from build123d import *

# Parameters (mm, degrees)
EXTRUDE023_DEPTH                          = 4
EXTRUDE022_DEPTH                          = 4
EXTRUDE022_ONTO_SKETCH021_PLACEMENT_ANGLE = 120


with BuildPart() as extrude023:
    # Sketch022 (on Face6 of Extrude022) → Extrude023 (new body)
    with BuildSketch(Plane(origin=(26.5, 0, 0), x_dir=(0, -1, 0), z_dir=(-1, 0, 0))):
        Polygon((-15.99404, 23.43698), (-11, 10), (-19, 10), (-22.458142, 20.240827), align=None)
    extrude(amount=-EXTRUDE023_DEPTH)


with BuildPart() as pin_boot:
    # Sketch021 as drawn → Extrude022 (new)
    with BuildSketch(Plane.XY):
        Polygon((29, 44.3), (33, 44.3), (33, 18.3), (30.5, 12.3), (30.5, 6.3), (26.5, 6.3), (26.5, 12.3), (29, 18.3), align=None)
    extrude(amount=EXTRUDE022_DEPTH)


with BuildPart() as pin_boot_1:
    # Extrude022 onto Sketch021 placement: moved
    add(pin_boot.part.moved(Location((0, 25.608142, 14.784867))).rotate(Axis((0, 25.608142, 14.784867), (1, 0, 0)), EXTRUDE022_ONTO_SKETCH021_PLACEMENT_ANGLE))

    # Connect005: union Extrude023
    add(extrude023.part)


solid = pin_boot_1.part
For this review, take the finished solid that the model builds, in its own axes (mm). A direction names the side the tool comes from. Give positions to 0.01 mm unless a question says otherwise; leave off trailing zeros. Loops run counter-clockwise (first coordinate to the right, second up) from the corner with the lowest first, then second, coordinate; pieces in that order, holes last. Notation, with made-up numbers: (-32, -7) -> (23, -7) arc R22 cw to (23, 15) -> close; hole circle Ø4 at (64.5, 67.5). An arc over 180 degrees is marked (long way). One line per question, with ' | ' between items.
1) We need section A-A (y = 11.5). Write out the cut boundary in (x, z), plus the area to 3 significant figures.
Resolved:
outline: (26.5, 10) -> (30.5, 10) -> (30.5, 11.35) -> (26.5, 11.35) -> close; (29, 31.22) -> (33, 31.22) -> (33, 39.22) -> (29, 39.22) -> close | area: 37.4 mm2
2) For faces 1 (the flat face through (28.47, 13.53, 16.81)), 2 (the flat face through (30.972, 1.75, 52.164)), list the 3-axis set-ups (+Z, -Z, +X, -X, +Y, -Y) from which the entire face can be reached by the end or side of a thin tool; tool diameter is ignored.
Resolved:
face 1: +X, -X, -Y | face 2: +Z, +X, -X, -Y
3) We need section C-C (z = 13.5). Write out the cut boundary in (x, y), plus the area to 3 significant figures.
Resolved:
outline: (26.5, 12.3) -> (30.5, 12.3) -> (30.5, 20.18) -> (26.5, 20.18) -> close | area: 31.5 mm2
4) We need section D-D (y = 5.5). Write out the cut boundary in (x, z).
Resolved:
outline: (29, 41.61) -> (33, 41.61) -> (33, 49.61) -> (29, 49.61) -> close
5) We need section B-B (x = 30). Write out the cut boundary in (y, z), plus the area to 3 significant figures.
Resolved:
outline: (-0.01, 51.15) -> (15.99, 23.44) -> (11, 10) -> (19, 10) -> (22.46, 20.24) -> (3.46, 53.15) -> close | area: 232 mm2
6) Insertion check: pin 1 Ø8 at (y, z) = (8.5, 39) entering from -X; pin 2 Ø1.5 at (x, z) = (27.5, 43) entering from -Y; pin 3 Ø5.5 at (y, z) = (16.5, 21) entering from +X; pin 4 Ø1.5 at (x, y) = (28, 18.5) entering from +Z. Each pin has a flat end and moves straight along its axis. Give the tip position at first contact, or say it passes through.
Resolved:
pin 1: stops at x = 29 | pin 2: passes through | pin 3: stops at x = 30.61 | pin 4: stops at z = 28.4
7) To check wall thickness, follow probe 1 along X at (y, z) = (20.5, 22); probe 2 along Y at (x, z) = (32.25, 49); probe 3 along Y at (x, z) = (32.5, 48). State the ranges of each line that lie inside material, in increasing order.
Resolved:
probe 1: x = 26.5 to 30.5 | probe 2: y = 1.24 to 5.85 | probe 3: y = 1.81 to 6.43
8) The part is to be moulded in two halves that separate along Z. For faces 3 (the flat face through (30.52, 7.88, 37.49)), 4 (the flat face through (28.472, 20.705, 15.049)), 5 (the flat face through (27.73, 16.27, 27.01)), 6 (the flat face through (33, 8, 41)), say which applies: +Z half, -Z half, draft (parallel to the pull), parting line (faces both ways), or undercut.
Resolved:
face 3: undercut | face 4: -Z half | face 5: +Z half | face 6: draft
